For this review, take the finished solid that the model builds, in its own axes (mm). A direction names the side the tool comes from. Give positions to 0.01 mm unless a question says otherwise; leave off trailing zeros. Write each loop counter-clockwise with the first axis right and the second up, starting at its lowest first coordinate (ties: lowest second). Pieces come first, ordered by that corner, then holes. Notation, with made-up numbers: (5.25, 18.5) -> (34.25, 18.5) arc R23 cw to (34.25, 41.5) -> close; hole circle Ø9 at (-12.75, 35.5). An arc over 180 degrees is marked (long way). Return JSON: item names as keys, results as strings.
Autodesk Inventor part; units mm, degrees
ref_plane "YZ Plane" through (0, 0, 0) normal (1, 0, 0) x (0, 1, 0)
ref_plane "XZ Plane" through (0, 0, 0) normal (0, 1, 0) x (-1, 0, 0)
ref_plane "XY Plane" through (0, 0, 0) normal (0, 0, 1) x (1, 0, 0)
sketch "Sketch1" plane through (0, 0, 0) normal (0, 0, 1) x (1, 0, 0)
  line L0 (0, 0) -> (48, 0)
  line L1 (48, 0) -> (48, 48)
  line L2 (48, 48) -> (0, 48)
  line L3 (0, 48) -> (0, 0)
  line L4 (10.5, 10.5) -> (5.5, 10.5)
  line L5 (5.5, 10.5) -> (5.5, 5.5)
  line L6 (5.5, 5.5) -> (10.5, 5.5)
  line L7 (10.5, 5.5) -> (10.5, 10.5)
  line L8 (10.5, 10.5) -> (5.5, 5.5) construction
  line L9 (5.5, 10.5) -> (10.5, 5.5) construction
  line L10 (5.5, 42.5) -> (10.5, 42.5)
  line L11 (10.5, 42.5) -> (10.5, 37.5)
  line L12 (10.5, 37.5) -> (5.5, 37.5)
  line L13 (5.5, 37.5) -> (5.5, 42.5)
  line L14 (5.5, 42.5) -> (10.5, 37.5) construction
  line L15 (10.5, 42.5) -> (5.5, 37.5) construction
  line L16 (42.5, 5.5) -> (37.5, 5.5)
  line L17 (37.5, 5.5) -> (37.5, 10.5)
  line L18 (37.5, 10.5) -> (42.5, 10.5)
  line L19 (42.5, 10.5) -> (42.5, 5.5)
  line L20 (42.5, 5.5) -> (37.5, 10.5) construction
  line L21 (37.5, 5.5) -> (42.5, 10.5) construction
  line L22 (42.5, 42.5) -> (37.5, 42.5)
  line L23 (37.5, 42.5) -> (37.5, 37.5)
  line L24 (37.5, 37.5) -> (42.5, 37.5)
  line L25 (42.5, 37.5) -> (42.5, 42.5)
  line L26 (42.5, 42.5) -> (37.5, 37.5) construction
  line L27 (37.5, 42.5) -> (42.5, 37.5) construction
  line L28 (37.5, 5.5) -> (37.5, 6.1)
  line L29 (37.5, 6.1) -> (10.5, 10.5)
  line L30 (37.5, 5.5) -> (10.5, 9.9)
  line L31 (37.5, 37.5) -> (37.5, 38.1)
  line L32 (37.5, 38.1) -> (10.5, 42.5)
  line L33 (37.5, 37.5) -> (10.5, 41.9)
  line L34 (0, 24) -> (0, 23.7)
  line L35 (0, 23.7) -> (48, 23.7)
  line L36 (48, 23.7) -> (48, 24.3)
  line L37 (48, 24.3) -> (0, 24.3)
  line L38 (0, 24.3) -> (0, 23.7)
  line L39 (5.5, 10.5) -> (6.1, 10.5)
  line L40 (6.1, 10.5) -> (6.1, 23.7)
  line L41 (6.1, 23.7) -> (5.5, 23.7)
  line L42 (5.5, 23.7) -> (5.5, 10.5)
  line L43 (10.5, 37.5) -> (9.9, 37.5)
  line L44 (9.9, 37.5) -> (9.9, 24.3)
  line L45 (9.9, 24.3) -> (10.5, 24.3)
  line L46 (10.5, 24.3) -> (10.5, 37.5)
  line L47 (37.5, 10.5) -> (38.1, 10.5)
  line L48 (38.1, 10.5) -> (38.1, 23.7)
  line L49 (38.1, 23.7) -> (37.5, 23.7)
  line L50 (37.5, 23.7) -> (37.5, 10.5)
  line L51 (42.5, 37.5) -> (41.9, 37.5)
  line L52 (41.9, 37.5) -> (41.9, 24.3)
  line L53 (41.9, 24.3) -> (42.5, 24.3)
  line L54 (42.5, 24.3) -> (42.5, 37.5)
  line L55 (10.5, 5.5) -> (9.9, 5.5)
  line L56 (9.9, 5.5) -> (9.9, 0)
  line L57 (9.9, 0) -> (10.5, 0)
  line L58 (10.5, 0) -> (10.5, 5.5)
  line L59 (42.5, 5.5) -> (41.9, 5.5)
  line L60 (41.9, 5.5) -> (41.9, 0)
  line L61 (41.9, 0) -> (42.5, 0)
  line L62 (42.5, 0) -> (42.5, 5.5)
  line L63 (37.5, 42.5) -> (38.1, 42.5)
  line L64 (38.1, 42.5) -> (38.1, 48)
  line L65 (38.1, 48) -> (37.5, 48)
  line L66 (37.5, 48) -> (37.5, 42.5)
  line L67 (5.5, 42.5) -> (6.1, 42.5)
  line L68 (6.1, 42.5) -> (6.1, 48)
  line L69 (6.1, 48) -> (5.5, 48)
  line L70 (5.5, 48) -> (5.5, 42.5)
  line L71 (5.5, 37.5) -> (0, 38.4621)
  line L72 (5.5, 37.5) -> (11.0835, 37.5) construction
  line L73 (5.5, 37.5) -> (5.5, 38.1)
  line L74 (5.5, 38.1) -> (0, 38.9963)
  line L75 (5.5, 5.5) -> (0, 6.4621)
  line L76 (5.5, 5.5) -> (11.0835, 5.5) construction
  line L77 (5.5, 5.5) -> (5.5, 6.1)
  line L78 (5.5, 6.1) -> (0, 6.9963)
  line L79 (42.5, 10.5) -> (48, 9.5379)
  line L80 (42.5, 10.5) -> (48.0835, 10.5) construction
  line L81 (42.5, 10.5) -> (42.5, 9.9)
  line L82 (42.5, 9.9) -> (48, 9.0037)
  line L83 (42.5, 42.5) -> (48, 41.6037)
  line L84 (42.5, 42.5) -> (42.5, 41.9)
  line L85 (42.5, 41.9) -> (48, 41.0037)
  line L86 (6.1, 24.3) -> (9.9, 24.3)
  line L87 (10.5, 24.3) -> (12.4, 24.3)
  arc A0 (12.4, 24.3) -> (8, 24.3) centre (10.2, 24.3124) ccw
  line L88 (5.5, 23.7) -> (3.6, 23.7)
  arc A1 (3.6, 23.7) -> (8, 23.7) centre (5.8, 23.7) ccw
  line L89 (41.9, 24.3) -> (40, 24.3)
  line L90 (42.5, 24.3) -> (44.4, 24.3)
  line L91 (37.5, 23.7) -> (35.6, 23.7)
  arc A2 (35.6, 23.7) -> (40, 23.7) centre (37.8, 23.7) ccw
  arc A3 (44.4, 24.3) -> (40, 24.3) centre (42.2, 24.3124) ccw
  point P0 (8, 24.3)
  point P1 (9.9, 26.4919)
  point P2 (41.9, 26.4919)
  point P3 (10.5, 26.4919)
  point P4 (42.5, 26.4919)
  point P5 (38.1, 21.5205)
  point P6 (37.5, 21.5206)
  point P7 (6.1, 21.5205)
  point P8 (5.5, 21.5206)
  dimension "d33" = 48
  dimension "d34" = 48
  dimension "d38" = 5
  dimension "d39" = 5
  dimension "d40" = 5
  dimension "d41" = 5
  dimension "d45" = 5
  dimension "d46" = 5
  dimension "d47" = 5
  dimension "d48" = 5
  dimension "d49" = 32
  dimension "d50" = 32
  dimension "d51" = 32
  dimension "d52" = 32
  dimension "d53" = 0.6
  dimension "d54" = 0.6
  dimension "d55" = 0.3
  dimension "d56" = 0.6
  dimension "d57" = 0.6
  dimension "d58" = 0.6
  dimension "d59" = 0.6
  dimension "d60" = 0.6
  dimension "d61" = 0.6
  dimension "d62" = 0.6
  dimension "d63" = 0.6
  dimension "d64" = 0.6
  dimension "d65" = 170.078
  dimension "d66" = 0.6
  dimension "d67" = 170.078
  dimension "d68" = 0.6
  dimension "d69" = 9.922
  dimension "d70" = 0.6
  dimension "d71" = 0.6
  dimension "d72" = 1.9
  dimension "d73" = 1.9
  dimension "d74" = 1.9
  dimension "d75" = 1.9
  dimension "d76" = 1.9
  dimension "d77" = 1.9
extrude "Extrusion1" add sketch "Sketch1" against normal blind 0.4 contours L3 L75 L6 L56 L0 | L58 L7 L30 L16 L60 L0 | L3 L35 A1 L42 L5 L78 | L62 L19 L82 L1 L0 | L4 L40 A1 L35 A2 L50 L17 L29 | L3 L71 L12 L44 A0 L37 | L79 L18 L48 A2 L35 L1 | L3 L2 L70 L13 L74 | L37 A3 L54 L25 L85 L1 | L11 L33 L24 L52 A3 L37 A0 L46 | L2 L66 L23 L32 L10 L68 | L83 L22 L64 L2 L1
extrude "Extrusion2" add sketch "Sketch1" along normal blind 1.6 contours L3 L75 L6 L56 L0 | L56 L6 L58 L0 | L3 L78 L5 L75 | L58 L7 L30 L16 L60 L0 | L3 L35 A1 L42 L5 L78 | L60 L16 L62 L0 | L3 L37 L1 L35 | L62 L19 L82 L1 L0 | L7 L29 L17 L30 | L35 L42 A1 | L42 A1 L40 L4 | L4 L40 A1 L35 A2 L50 L17 L29 | L3 L71 L12 L44 A0 L37 | L35 L40 A1 L42 | L82 L19 L79 L1 | L3 L74 L13 L71 | L35 A1 L40 | L79 L18 L48 A2 L35 L1 | L50 A2 L48 L18 | L3 L2 L70 L13 L74 | A0 L44 L37 | A2 L35 L50 | L50 L35 L48 A2 | L12 L46 A0 L44 | L44 A0 L46 L37 | L37 A3 L54 L25 L85 L1 | A2 L48 L35 | L2 L68 L10 L70 | L11 L33 L24 L52 A3 L37 A0 L46 | L46 A0 L37 | L85 L25 L83 L1 | L37 L54 A3 | L2 L66 L23 L32 L10 L68 | L11 L32 L23 L33 | L83 L22 L64 L2 L1 | L37 L52 A3 L54 | A3 L52 L24 L54 | L2 L64 L22 L66 | A3 L52 L37
properties part number "LED Position"
1. For faces 1 (the flat face through (22, 44, -0.4)), 2 (the flat face through (45.2, 9.8, 0)), 3 (the flat face through (8, 37.5, 1)), list the 3-axis set-ups (+Z, -Z, +X, -X, +Y, -Y) from which the entire face can be reached by the end or side of a thin tool; tool diameter is ignored.
Results found:
{"face 1": "-Z, +X, -X, +Y, -Y", "face 2": "-Z", "face 3": "+Z, -Z"}
2. The part is to be moulded in two halves that separate along Y. For faces 4 (the flat face through (5, 3, -0.4)), 5 (the flat face through (40, 5.5, 1)), 6 (the flat face through (24, 0, 1)), say which applies: +Y half, -Y half, draft (parallel to the pull), parting line (faces both ways), or undercut.
Results found:
{"face 4": "draft", "face 5": "undercut", "face 6": "-Y half"}
3. Add section A-A, the plane z = 1.25. State the section outline as (x, y) points.
Results found:
{"outline": "(0, 0) -> (48, 0) -> (48, 48) -> (0, 48) -> close; hole (5.5, 5.5) -> (10.5, 5.5) -> (10.5, 10.5) -> (5.5, 10.5) -> close; hole (5.5, 37.5) -> (10.5, 37.5) -> (10.5, 42.5) -> (5.5, 42.5) -> close; hole (37.5, 5.5) -> (42.5, 5.5) -> (42.5, 10.5) -> (37.5, 10.5) -> close; hole (37.5, 37.5) -> (42.5, 37.5) -> (42.5, 42.5) -> (37.5, 42.5) -> close"}
4. Add section B-B, the plane x = 39. State the section outline as (y, z) points.
Results found:
{"outline": "(0, -0.4) -> (5.5, -0.4) -> (5.5, 1.6) -> (0, 1.6) -> close; (10.5, -0.4) -> (21.86, -0.4) -> (21.86, 0) -> (24.3, 0) -> (24.3, -0.4) -> (37.5, -0.4) -> (37.5, 1.6) -> (10.5, 1.6) -> close; (42.5, -0.4) -> (48, -0.4) -> (48, 1.6) -> (42.5, 1.6) -> close"}
5. To check wall thickness, follow probe 1 along X at (y, z) = (7, 1.1); probe 2 along Y at (x, z) = (39.5, -0.1). State the ranges of each line that lie inside material, in increasing order.
Results found:
{"probe 1": "x = 0 to 5.5, 10.5 to 37.5, 42.5 to 48", "probe 2": "y = 0 to 5.5, 10.5 to 22.3, 24.3 to 37.5, 42.5 to 48"}
